```python
from build123d import *

# Parameters (mm, degrees)
SKETCH_2_R          = 4.5
EXTRUDE_1_DEPTH     = 10
EXTRUDE_2_DEPTH     = 4
SKETCH_5_R          = 3
EXTRUDE_3_DEPTH     = 2
SKETCH_6_R          = 0.9
CUT_EXTRUDE_1_DEPTH = 8
SKETCH_7_R          = 2.5
EXTRUDE_4_DEPTH     = 5


with BuildPart() as part:
    # 草图2 → 凸台-拉伸1 (new body)
    with BuildSketch(Plane.XY):
        with BuildLine():
            Line((7.102160211, -15.616687508), (44.391240582, 21.672392863))
            ThreePointArc((44.391240582, 21.672392863), (45.562813457, 24.500819988), (44.391240582, 27.329247112))
            Line((44.391240582, 27.329247112), (34.138192255, 37.58229544))
            ThreePointArc((34.138192255, 37.58229544), (31.30976513, 38.753868315), (28.481338005, 37.58229544))
            Line((28.481338005, 37.58229544), (9.215390399, 18.316347834))
            ThreePointArc((9.215390399, 18.316347834), (8.067593218, 16.131525495), (8.362136672, 13.681192624))
            ThreePointArc((8.362136672, 13.681192624), (9.134610316, 6.948541986), (5.886174479, 1.001024456))
            ThreePointArc((5.886174479, 1.001024456), (-7.225109998, -13.84439598), (-17.685225472, -30.663381468))
            ThreePointArc((-17.685225472, -30.663381468), (-11.168239652, -44.207967845), (0.129369861, -34.293788928))
            ThreePointArc((0.129369861, -34.293788928), (1.585802578, -24.197384934), (7.102160211, -15.616687508))
        make_face()
        with Locations((-9.283850525, -34.961173895)):
            Circle(SKETCH_2_R, mode=Mode.SUBTRACT)
        Polygon((39.229361079, 23.581581172), (22.6830624, 7.035282492), (13.844227635, 15.874117257), (30.390526315, 32.420415937), align=None, mode=Mode.SUBTRACT)
    extrude(amount=EXTRUDE_1_DEPTH)

    # 草图4 → 凸台-拉伸2 (add, symmetric)
    with BuildSketch(Plane(origin=(3.298406554, -3.298406554, 0), x_dir=(0, 0, -1), z_dir=(0.7071067811865492, -0.7071067811865458, 0))):
        with BuildLine():
            Line((0, 49.014043199), (0, 46.014043199))
            Line((0, 46.014043199), (7, 46.014043199))
            Line((7, 46.014043199), (7, 20.014043199))
            Line((7, 20.014043199), (0, 20.014043199))
            Line((0, 20.014043199), (0, 17.014043199))
            Line((0, 17.014043199), (8, 17.014043199))
            ThreePointArc((8, 17.014043199), (10.828427125, 18.185616074), (12, 21.014043199))
            Line((12, 21.014043199), (12, 45.014043199))
            ThreePointArc((12, 45.014043199), (10.828427125, 47.842470323), (8, 49.014043199))
            Line((8, 49.014043199), (0, 49.014043199))
        make_face()
    extrude(amount=EXTRUDE_2_DEPTH, both=True)

    # 草图5 → 凸台-拉伸3 (add)
    with BuildSketch(Plane(origin=(0, 0, -12), x_dir=(-1, 0, 0), z_dir=(0, 0, -1))):
        with Locations((-30.461236993, 23.864423885)):
            Circle(SKETCH_5_R)
    extrude(amount=EXTRUDE_3_DEPTH)

    # 草图6 → 切除-拉伸1 (cut)
    with BuildSketch(Plane.XY.offset(10)):
        with Locations((16.354456708, 9.7576436)):
            Circle(SKETCH_6_R)
        with Locations((36.506999972, 29.910186864)):
            Circle(SKETCH_6_R)
    extrude(amount=-CUT_EXTRUDE_1_DEPTH, mode=Mode.SUBTRACT)

    # 草图7 → 凸台-拉伸4 (add)
    with BuildSketch(Plane(origin=(0, 0, -14), x_dir=(-1, 0, 0), z_dir=(0, 0, -1))):
        with Locations((-30.461236993, 23.864423885)):
            Circle(SKETCH_7_R)
    extrude(amount=EXTRUDE_4_DEPTH)


solid = part.part
```
Source: CAD feature listing. Evaluate the final solid. Frame: model axes, mm. A direction names the side the tool comes from. Give positions to 0.01 mm unless a question says otherwise; leave off trailing zeros. Loops run counter-clockwise (first coordinate to the right, second up) from the corner with the lowest first, then second, coordinate; pieces in that order, holes last. Notation, with made-up numbers: (2.5, -11.5) -> (39.5, -11.5) arc R23 cw to (39.5, 20.5) -> close; hole circle Ø6 at (3.5, 47). An arc over 180 degrees is marked (long way). Use a Markdown table: item, result. Add a question column.
(1) First-contact query: pin 1 Ø7 at (x, y) = (-9.28, -34.96) entering from -Z; pin 2 Ø5 at (x, z) = (11, 2) entering from +Y; pin 3 Ø1.5 at (y, z) = (14, 6) entering from +X; pin 4 Ø0.9 at (x, y) = (36.5, 29.5) entering from +Z. Flat tips, straight axial feed; report the tip coordinate or a pass-through.
(2) Section query C-C (y = 0). Output: boundary loops of the cut face in (x, z).
(3) Section query B-B (z = 4.5). Output: boundary loops of the cut face in (x, y), then the cut area to 3 significant figures.
(4) Pull-direction query (X, two-part tool) for faces 5 (the face through (19, 28.1, 4.9)), 6 (the face through (17.213, 10.028, 6.056)), 7 (the face through (31.354, 38.754, 4.93)), 8 (the face through (37.146, 30.47, -10.859)); classes: +X half, -X half, draft (parallel to the pull), parting line (faces both ways), or undercut.
(5) Section query A-A (z = -5.75). Output: boundary loops of the cut face in (x, y) (3 decimals).
(6) Section query D-D (z = -15.75). Output: boundary loops of the cut face in (x, y), then the cut area to 3 significant figures.
(7) Access query for faces 1 (the face through (15.37, 8.69, -3.94)), 2 (the face through (33.46, 24, -12.99)), 3 (the face through (22, 24.03, 4.93)), 4 (the face through (17.49, 10.814, -3.549)). Directions: +Z, -Z, +X, -X, +Y, -Y. A direction counts if a zero-diameter tool reaches every point of the face in a straight line with its end or side. Return the directions, or none.
(8) Ray query, line 1 (X direction, y = 13, z = 1); line 2 (Z direction, x = 3.5, y = -12); line 3 (X direction, y = 28, z = 5.25). Return the intervals inside material, ascending.
Checked values:
| question | item | result |
|---|---|---|
| 1 | pin 1 | through |
| 1 | pin 2 | y = 22.6 |
| 1 | pin 3 | x = 37.47 |
| 1 | pin 4 | z = 2 |
| 2 | outline | (4.85, 0) -> (22.72, 0) -> (22.72, 10) -> (4.85, 10) -> close |
| 3 | outline | (-17.69, -30.66) arc R9.44 ccw (long way) to (0.13, -34.29) arc R24.01 cw to (7.1, -15.62) -> (44.39, 21.67) arc R4 ccw to (44.39, 27.33) -> (34.14, 37.58) arc R4 ccw to (28.48, 37.58) -> (9.22, 18.32) arc R4.15 ccw to (8.36, 13.68) arc R11.21 cw to (5.89, 1) arc R118.69 ccw to start; hole circle Ø9 at (-9.28, -34.96); hole (13.84, 15.87) -> (22.68, 7.04) -> (39.23, 23.58) -> (30.39, 32.42) -> close; hole circle Ø1.8 at (16.35, 9.76); hole circle Ø1.8 at (36.51, 29.91) |
| 3 | area | 1,240 mm^2 |
| 4 | face 5 | -X half |
| 4 | face 6 | undercut |
| 4 | face 7 | parting line |
| 4 | face 8 | +X half |
| 5 | outline | (12.501, 11.561) -> (18.158, 5.904) -> (20.279, 8.025) -> (14.622, 13.682) -> close; (33.007, 32.067) -> (38.664, 26.41) -> (40.785, 28.531) -> (35.128, 34.188) -> close |
| 6 | outline | circle Ø5 at (30.46, 23.86) |
| 6 | area | 19.6 mm^2 |
| 7 | face 1 | -Z, -X, -Y |
| 7 | face 2 | -Z |
| 7 | face 3 | +Z, -Z |
| 7 | face 4 | +X, +Y |
| 8 | line 1 | 8.64 to 16.72, 28.65 to 35.72 |
| 8 | line 2 | 0 to 10 |
| 8 | line 3 | 18.9 to 25.97, 34.81 to 43.72 |
